Autodesk Inventor part; units mm, degrees
ref_plane "YZ Plane (RIGHT)" through (0, 0, 0) normal (1, 0, 0) x (0, 1, 0)
ref_plane "XZ Plane (TOP)" through (0, 0, 0) normal (0, 1, 0) x (-1, 0, 0)
ref_plane "XY Plane (FRONT)" through (0, 0, 0) normal (0, 0, 1) x (1, 0, 0)
sketch "Sketch2" plane through (0, 0, 0) normal (0, 0, 1) x (1, 0, 0)
  line L0 (-4.445, 0) -> (4.445, 0) construction
  line L1 (0, 9.8146) -> (0, -1.6358) construction
  line L2 (-3.175, 0) -> (3.175, 0)
  line L3 (2.159, 3.175) -> (-3.175, 3.175)
  line L4 (-3.175, 3.175) -> (-3.175, 0)
  line L5 (3.175, 0) -> (3.175, 8.1788)
  line L6 (3.175, 8.1788) -> (2.159, 8.1788)
  line L7 (2.159, 8.1788) -> (1.4478, 6.5607)
  line L8 (1.4478, 6.5607) -> (2.159, 4.9425)
  line L9 (2.159, 4.9425) -> (2.159, 3.175)
  point P0 (0, 0)
  dimension "d0" = 6.35
  dimension "d1" = 3.175
  dimension "d2" = 8.1788
  dimension "d3" = 1.4478
  dimension "d4" = 1.016
extrude "Extrusion1" add sketch "Sketch2" along normal mid plane 2.54
sketch "Sketch3" plane through (-3.175, 0, 1.27) normal (0, -1, 0) x (1, 0, 0)
  line L0 (-1.27, -1.27) -> (7.62, -1.27) construction
  line L1 (3.175, 0.508) -> (3.175, -3.048) construction
  line L2 (2.794, -0.889) -> (3.556, -0.889)
  line L3 (3.556, -0.889) -> (3.556, -1.651)
  line L4 (3.556, -1.651) -> (2.794, -1.651)
  line L5 (2.794, -1.651) -> (2.794, -0.889)
  circle A0 centre (3.175, -1.27) radius 0.4445
  dimension "d7" = 0.762
  dimension "d15" = 0.889
extrude "Extrusion2" add sketch "Sketch3" along normal blind 3.556 contours A0 L2 | L2 A0 L3 L4 L5 | L5 A0 | A0 L3 | L4 A0
extrude "Extrusion3" add sketch "Sketch3" against normal blind 10.668 contours L2 A0 L5 | L2 A0 L3 L4 L5 | L2 L3 A0 | A0 L4 L5 | L3 L4 A0
pattern_linear "Rectangular Pattern1" count 3 spacing 2.54 along (0, 0, 1) of "Extrusion1", "Extrusion2", "Extrusion3"
properties part number "Molex KK 3 Pin"
Source: CAD feature listing. Evaluate the final solid. Frame: model axes, mm. A direction names the side the tool comes from. Give positions to 0.01 mm unless a question says otherwise; leave off trailing zeros. Write each loop counter-clockwise with the first axis right and the second up, starting at its lowest first coordinate (ties: lowest second). Pieces come first, ordered by that corner, then holes. Notation, with made-up numbers: (51, 24) -> (88, 24) arc R26 ccw to (88, 54) -> close; hole circle Ø8 at (-26.75, 45.5). An arc over 180 degrees is marked (long way). Return JSON: item names as keys, results as strings. Group by question number.
1. Material intervals for line 1 (X direction, y = 3.75, z = 2.5) (3 decimals); line 2 (Z direction, x = 0, y = 7); line 3 (Y direction, x = 1, z = 6) (3 decimals), sorted ascending. Write a range as from..to.
2. Section B-B, the plane z = 2.54. Output: boundary loops of the cut face in (x, y) (1 decimal).
3. Access query for faces 4 (the face through (1.8, 5.76, 2.49)), 5 (the face through (3, 8.179, 2)), 6 (the face through (1, 2, -1.27)), 7 (the face through (-0.096, -1.753, 5.514)), 8 (the face through (1.81, 7.38, 2.49)). Directions: +Z, -Z, +X, -X, +Y, -Y. A direction counts if a zero-diameter tool reaches every point of the face in a straight line with its end or side. Return the directions, or none.
4. Pin query (flat end, axial travel): pin 1 Ø0.8 at (y, z) = (8.5, 0) entering from -X; pin 2 Ø3 at (x, z) = (0, 4) entering from +Y; pin 3 Ø0.8 at (x, y) = (0, 8) entering from +Z; pin 4 Ø0.5 at (x, z) = (3, 1.5) entering from +Y. Return the tip coordinate at first contact, or that it passes through.
5. Mould query, pull axis Z, two halves, no side actions, for faces 1 (the face through (-0.096, -1.753, 0.434)), 2 (the face through (1, 2, 6.35)), 3 (the face through (0, -3.556, 0)). Classes: +Z half, -Z half, draft (parallel to the pull), parting line (faces both ways), or undercut.
6. Section D-D, the plane y = 5.5. Output: boundary loops of the cut face in (x, z) (3 decimals), then the cut area to 3 significant figures.
7. Section A-A, the plane y = 4. Output: boundary loops of the cut face in (x, z) (3 decimals), then the cut area to 3 significant figures.
Determined:
{
 "1": {"line 1": "x = -0.381..0.381, 2.159..3.175", "line 2": "z = -0.38..0.38, 2.16..2.92, 4.7..5.46", "line 3": "y = 0..3.175"},
 "2": {"outline": "(-3.2, 0) -> (-0.4, 0) -> (-0.4, -3.6) -> (0.4, -3.6) -> (0.4, 0) -> (3.2, 0) -> (3.2, 8.2) -> (2.2, 8.2) -> (1.4, 6.6) -> (2.2, 4.9) -> (2.2, 3.2) -> (0.4, 3.2) -> (0.4, 10.7) -> (-0.4, 10.7) -> (-0.4, 3.2) -> (-3.2, 3.2) -> close"},
 "3": {"face 4": "+Z, -Z", "face 5": "+Z, -Z, +X, +Y", "face 6": "-Z, +X, -X, +Y, -Y", "face 7": "-Y", "face 8": "+Z, -Z, +Y"},
 "4": {"pin 1": "stops at x = -0.38", "pin 2": "stops at y = 10.67", "pin 3": "stops at z = 5.46", "pin 4": "stops at y = 8.18"},
 "5": {"face 1": "undercut", "face 2": "+Z half", "face 3": "draft"},
 "6": {"outline": "(-0.381, -0.381) -> (0.381, -0.381) -> (0.381, 0.381) -> (-0.381, 0.381) -> close; (-0.381, 2.159) -> (0.381, 2.159) -> (0.381, 2.921) -> (-0.381, 2.921) -> close; (-0.381, 4.699) -> (0.381, 4.699) -> (0.381, 5.461) -> (-0.381, 5.461) -> close; (1.914, -1.27) -> (3.175, -1.27) -> (3.175, 6.35) -> (1.914, 6.35) -> close", "area": "11.4 mm2"},
 "7": {"outline": "(-0.381, -0.381) -> (0.381, -0.381) -> (0.381, 0.381) -> (-0.381, 0.381) -> close; (-0.381, 2.159) -> (0.381, 2.159) -> (0.381, 2.921) -> (-0.381, 2.921) -> close; (-0.381, 4.699) -> (0.381, 4.699) -> (0.381, 5.461) -> (-0.381, 5.461) -> close; (2.159, -1.27) -> (3.175, -1.27) -> (3.175, 6.35) -> (2.159, 6.35) -> close", "area": "9.48 mm2"}
}
